Check sheet for the drawn part. Datum: minimum x, y, z corner. Units: mm. A direction names the side the tool comes from. Coordinates: 2 decimals unless noted, no trailing zeros. Write each loop counter-clockwise with the first axis right and the second up, starting at its lowest first coordinate (ties: lowest second). Pieces come first, ordered by that corner, then holes. Notation, with made-up numbers: (-7, -27.5) - (2, -27.5) arc R16 cw to (2, -20.5) - close; hole circle Ø3 at (53.5, -1). An arc over 180 degrees is marked (long way). Answer as CSV lines item,"result". Start each with the question number.
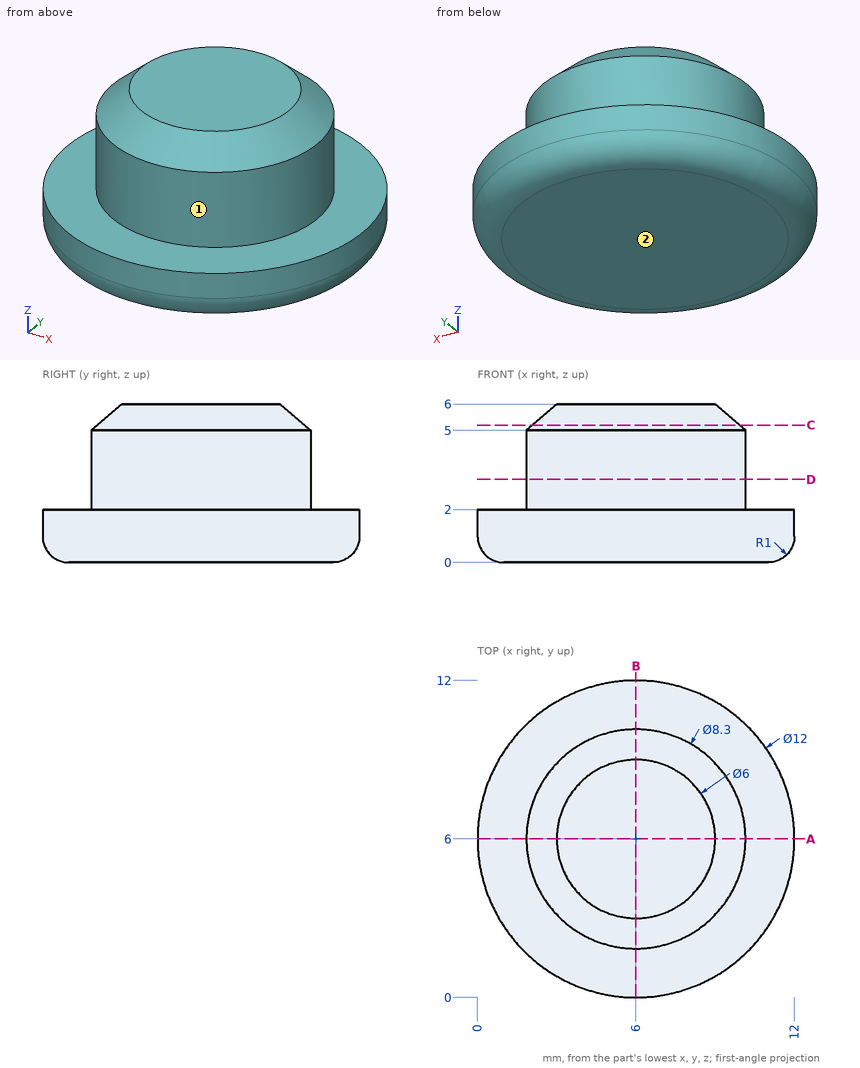
(1) Cross-section at A-A on y = 6. Record the boundary of the cut face in (x, z), plus the area to 3 significant figures.
(2) Material ranges on probe 1 along Z at (x, y) = (2, 4.25); probe 2 along X at (y, z) = (9.25, 2.2); probe 3 along X at (y, z) = (9.75, 2.95), recorded low to high. Write a range as from..to.
(3) Cross-section at C-C on z = 5.2. Record the boundary of the cut face in (x, y).
(4) Cross-section at D-D on z = 3.15. Record the boundary of the cut face in (x, y), plus the area to 3 significant figures.
(5) Tool access check on the marked faces 1 and 2. Record the directions out of +Z, -Z, +X, -X, +Y, -Y that give a thin tool (end or side, any length) a straight path to the whole face; none if there is none.
Checked values:
1,outline,"(0, 1) arc R1 ccw to (1, 0) - (11, 0) arc R1 ccw to (12, 1) - (12, 2) - (10.15, 2) - (10.15, 5) - (9, 6) - (3, 6) - (1.85, 5) - (1.85, 2) - (0, 2) - close"
1,area,"55.6 mm^2"
2,probe 1,"0..2"
2,probe 2,"3.42..8.58"
2,probe 3,"4.22..7.78"
3,outline,"circle Ø7.84 at (6, 6)"
4,outline,"circle Ø8.3 at (6, 6)"
4,area,"54.1 mm^2"
5,face 1,"+Z"
5,face 2,"-Z, +X, -X, +Y, -Y"
